```python
from build123d import *

# Parameters (mm, degrees)
SKETCH2_R           = 25
SKETCH2_R_2         = 5.25
SKETCH2_R_3         = 1.75
BOSS_EXTRUDE1_DEPTH = 2.825
SKETCH3_R           = 16.125
SKETCH3_R_2         = 7.875
CUT_EXTRUDE1_DEPTH  = 3


with BuildPart() as part:
    # Sketch2 → Boss-Extrude1 (new, symmetric)
    with BuildSketch(Plane(origin=(0, 0, 0), x_dir=(1, 0, 0), z_dir=(0, 1, 0))):
        with Locations(Location((0, 0, 0), (0, 0, 270))):
            Circle(SKETCH2_R)
        with Locations(Location((0, 0, 0), (0, 0, 270))):
            Circle(SKETCH2_R_2, mode=Mode.SUBTRACT)
        with Locations(Location((0, 21.25, 0), (0, 0, 270))):
            Circle(SKETCH2_R_3, mode=Mode.SUBTRACT)
        with Locations(Location((15.0260191, 15.0260191, 0), (0, 0, 270))):
            Circle(SKETCH2_R_3, mode=Mode.SUBTRACT)
        with Locations(Location((21.25, 0, 0), (0, 0, 270))):
            Circle(SKETCH2_R_3, mode=Mode.SUBTRACT)
        with Locations(Location((15.0260191, -15.0260191, 0), (0, 0, 270))):
            Circle(SKETCH2_R_3, mode=Mode.SUBTRACT)
        with Locations(Location((0, -21.25, 0), (0, 0, 270))):
            Circle(SKETCH2_R_3, mode=Mode.SUBTRACT)
        with Locations(Location((-15.0260191, -15.0260191, 0), (0, 0, 270))):
            Circle(SKETCH2_R_3, mode=Mode.SUBTRACT)
        with Locations(Location((-21.25, 0, 0), (0, 0, 270))):
            Circle(SKETCH2_R_3, mode=Mode.SUBTRACT)
        with Locations(Location((-15.0260191, 15.0260191, 0), (0, 0, 270))):
            Circle(SKETCH2_R_3, mode=Mode.SUBTRACT)
    extrude(amount=BOSS_EXTRUDE1_DEPTH, both=True)

    # Sketch3 → Cut-Extrude1 (cut)
    with BuildSketch(Plane(origin=(0, 2.825, 0), x_dir=(1, 0, 0), z_dir=(0, 1, 0))):
        with Locations(Location((0, 0, 0), (0, 0, 270))):
            Circle(SKETCH3_R)
        with Locations(Location((0, 0, 0), (0, 0, 270))):
            Circle(SKETCH3_R_2, mode=Mode.SUBTRACT)
    extrude(amount=-CUT_EXTRUDE1_DEPTH, mode=Mode.SUBTRACT)


solid = part.part
```
Check sheet for the modelled part. Datum: model origin and axes. Units: mm. A direction names the side the tool comes from. Coordinates: 2 decimals unless noted, no trailing zeros. Write each loop counter-clockwise with the first axis right and the second up, starting at its lowest first coordinate (ties: lowest second). Pieces come first, ordered by that corner, then holes. Notation, with made-up numbers: M -10,-24.5 L 37,-24.5 A28 ccw 37,1.5 Z; hole C 28.25,36.25 d4. An arc over 180 degrees is marked long. Write item = value, one per line. Start each with the question number.
1. Sectioned sample at C-C (y = 0.5). State how many separate pieces and enclosed holes the cut face has, then the cut area to 3 significant figures.
2. Sectioned sample at A-A (x = 0). Record the cut outline in (y, z) (3 decimals).
3. Go/stop test with flat-tipped pins: pin 1 (3 mm diameter, centred on x = -21.25, z = 0, fed in from -Y); pin 2 (5.5 mm diameter, centred on x = -15.03, z = 15.03, fed in from -Y) (3 decimals); pin 3 (2 mm diameter, centred on y = -1.5, z = -7, fed in from +X). Record where each tip stops, or that it passes through.
4. Thickness scan on probe 1 along X at (y, z) = (-0.75, 0); probe 2 along X at (y, z) = (0.85, 0) (3 decimals); probe 3 along X at (y, z) = (0.2, -5.5). Record the ranges inside material, lowest first.
5. Sectioned sample at D-D (x = 21.25). Record the cut outline in (y, z) (3 decimals).
6. Mould release check, pull along X, two halves, no side actions. Record for faces 3 (the flat face through (1.9, 2.825, 5.1)), 4 (the cylindrical face through (-16.58, -0.04, -14.22)), 5 (the cylindrical face through (7.509, 0.04, 23.846)): pulls with the +X half, pulls with the -X half, needs draft (parallel to the pull), parting line crosses it, or undercut.
7. Sectioned sample at B-B (z = 0). Record the cut outline in (x, y) (3 decimals), then the cut area to 3 significant figures.
8. Tool access check on faces 1 (the cylindrical face through (4.84, 1.35, 15.38)), 2 (the cylindrical face through (0.08, -0.04, 19.5)). Record the directions out of +Z, -Z, +X, -X, +Y, -Y that give a thin tool (end or side, any length) a straight path to the whole face; none if there is none.
The answers:
q1.separate_pieces = 2
q1.enclosed_holes = 10
q1.area = 1,180 mm²
q2.outline = M -2.825,-25 L 2.825,-25 L 2.825,-23 L -2.825,-23 Z; M -2.825,-19.5 L 2.825,-19.5 L 2.825,-16.125 L -0.175,-16.125 L -0.175,-7.875 L 2.825,-7.875 L 2.825,-5.25 L -2.825,-5.25 Z; M -2.825,5.25 L 2.825,5.25 L 2.825,7.875 L -0.175,7.875 L -0.175,16.125 L 2.825,16.125 L 2.825,19.5 L -2.825,19.5 Z; M -2.825,23 L 2.825,23 L 2.825,25 L -2.825,25 Z
q3.pin_1 = through
q3.pin_2 = -2.825
q3.pin_3 = 24.27
q4.probe_1 = -25 to -23, -19.5 to -5.25, 5.25 to 19.5, 23 to 25
q4.probe_2 = -25 to -23, -19.5 to -16.125, -7.875 to -5.25, 5.25 to 7.875, 16.125 to 19.5, 23 to 25
q4.probe_3 = -24.39 to -15.16, -5.64 to 5.64, 15.16 to 24.39
q5.outline = M -2.825,-13.17 L 2.825,-13.17 L 2.825,-1.75 L -2.825,-1.75 Z; M -2.825,1.75 L 2.825,1.75 L 2.825,13.17 L -2.825,13.17 Z
q6.face_3 = needs draft
q6.face_4 = undercut
q6.face_5 = parting line crosses it
q7.outline = M -25,-2.825 L -23,-2.825 L -23,2.825 L -25,2.825 Z; M -19.5,-2.825 L -5.25,-2.825 L -5.25,2.825 L -7.875,2.825 L -7.875,-0.175 L -16.125,-0.175 L -16.125,2.825 L -19.5,2.825 Z; M 5.25,-2.825 L 19.5,-2.825 L 19.5,2.825 L 16.125,2.825 L 16.125,-0.175 L 7.875,-0.175 L 7.875,2.825 L 5.25,2.825 Z; M 23,-2.825 L 25,-2.825 L 25,2.825 L 23,2.825 Z
q7.area = 134 mm²
q8.face_1 = +Y
q8.face_2 = +Y, -Y
